Input: part model. Units: mm. Frame: model coordinates. Face numbers are marked on the shaded views. A direction names the side the tool comes from. Give positions to 0.01 mm unless a question says otherwise; leave off trailing zeros. Loops run counter-clockwise (first coordinate to the right, second up) from the corner with the lowest first, then second, coordinate; pieces in that order, holes last. Notation, with made-up numbers: M -5,-22 L 50,-22 A19 cw 50,0 Z; hole C 25.25,-2 d10. An arc over 180 degrees is marked long. Answer as a JSON object with one key per item and string values. Group by question number.
```python
from build123d import *

# Parameters (mm, degrees)
F0_R            = 5
F1_DEPTH        = 3
F3_D            = 2.4
F3_CBORE_D      = 4.4
F3_CBORE_DEPTH  = 2
F3_COPIES_COUNT = 3


# Not quite as in the source:
# - a pattern or mirror of a feature is missing from the dataset's text; its kind, count and spacing are read off the source's solid


with BuildPart() as f1:
    # F0 (on Top) → F1 (new body)
    with BuildSketch(Plane.XY):
        with BuildLine():
            Line((11.3, 4), (13.416407865, 4))
            ThreePointArc((13.416407865, 4), (-14, 0), (13.416407865, -4))
            Line((13.416407865, -4), (11.3, -4))
            Line((11.3, -4), (11.3, 4))
        make_face()
        Circle(F0_R, mode=Mode.SUBTRACT)
    extrude(amount=F1_DEPTH)

    # F3 (through all)
    with Locations(Plane.XY.offset(3)):
        with Locations((0, 11)):
            f3 = CounterBoreHole(F3_D / 2, F3_CBORE_D / 2, F3_CBORE_DEPTH)

    # F3_copies: F3 ×3 about axis
    f3_copies_axis = Axis((0, 0, 0), (0, 0, 1))
    for i in range(1, F3_COPIES_COUNT):
        add(f3.rotate(f3_copies_axis, i * 360 / F3_COPIES_COUNT), mode=Mode.SUBTRACT)


solid = f1.part
```
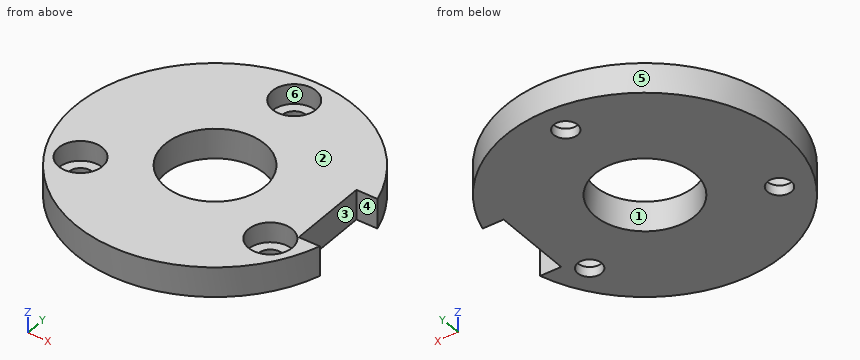
1. Reachability of the marked faces 4, 5 and 6 from +Z, -Z, +X, -X, +Y, -Y: full face, straight path, thin tool, end or side. Return the list, or none.
2. First-contact query: P1, Ø2, axis at x = 1, y = 11, coming from the +Z side; P2, Ø6, axis at x = 1.5, y = 3.5, coming from the +Z side; P3, Ø1.7, axis at x = 12, z = 1, coming from the +Y side; P4, Ø1.5, axis at x = -1, z = 2, coming from the +Y side. Flat tips, straight axial feed; report the tip coordinate or a pass-through.
3. Section C-C (x = -3). Output: boundary loops of the cut face in (y, z).
4. Section D-D (y = -5.5). Output: boundary loops of the cut face in (x, z), then the cut area to 3 significant figures.
5. Section B-B (x = 0). Output: boundary loops of the cut face in (y, z), then the cut area to 3 significant figures.
6. Mould query, pull axis X, two halves, no side actions, for the marked faces 1, 2 and 3. Classes: pulls with the +X half, pulls with the -X half, needs draft (parallel to the pull), parting line crosses it, or undercut.
7. Section A-A (y = 0). Output: boundary loops of the cut face in (x, z).
8. Material intervals for L1, parallel to Y at x = 0, z = 2.5; L2, parallel to Y at x = 1.5, z = 2.1; L3, parallel to X at y = -6, z = 0.65, sorted ascending.
Geometry results:
{
 "1": {"face 4": "+Z, -Z, +X", "face 5": "+Z, -Z", "face 6": "+Z"},
 "2": {"P1": "z = 1", "P2": "z = 3", "P3": "y = 8.47", "P4": "y = 14"},
 "3": {"outline": "M -13.67,0 L -4,0 L -4,3 L -13.67,3 Z; M 4,0 L 13.67,0 L 13.67,3 L 4,3 Z"},
 "4": {"outline": "M -12.87,0 L -10.73,0 L -10.73,1 L -11.73,1 L -11.73,3 L -12.87,3 Z; M -8.33,0 L 8.33,0 L 8.33,1 L 7.33,1 L 7.33,3 L -7.33,3 L -7.33,1 L -8.33,1 Z; M 10.73,0 L 12.87,0 L 12.87,3 L 11.73,3 L 11.73,1 L 10.73,1 Z", "area": "54.8 mm2"},
 "5": {"outline": "M -14,0 L -5,0 L -5,3 L -14,3 Z; M 5,0 L 9.8,0 L 9.8,1 L 8.8,1 L 8.8,3 L 5,3 Z; M 12.2,0 L 14,0 L 14,3 L 13.2,3 L 13.2,1 L 12.2,1 Z", "area": "42.8 mm2"},
 "6": {"face 1": "undercut", "face 2": "needs draft", "face 3": "pulls with the +X half"},
 "7": {"outline": "M -14,0 L -5,0 L -5,3 L -14,3 Z; M 5,0 L 11.3,0 L 11.3,3 L 5,3 Z"},
 "8": {"L1": "-14 to -5, 5 to 8.8, 13.2 to 14", "L2": "-13.92 to -4.77, 4.77 to 9.39, 12.61 to 13.92", "L3": "-12.65 to -10.62, -8.44 to 8.44, 10.62 to 12.65"}
}
